Could you check a few things on this model? Use its own coordinates, in mm. A direction names the side the tool comes from. Coordinates: 2 decimals unless noted, no trailing zeros. Loops run counter-clockwise (first coordinate to the right, second up) from the corner with the lowest first, then second, coordinate; pieces in that order, holes last.
from build123d import *

# Parameters (mm, degrees)
SKETCH_2_W               = 1.2
SKETCH_2_H               = 0.55
CHAMFER_1_SIZE           = 1
FILLET_1_R               = 0.4
HOLE_WIZARD_1_D          = 3
HOLE_WIZARD_1_DEPTH      = 15
PATTERN_CIRCULAR_1_COUNT = 4
SKETCH_5_W               = 2.5
SKETCH_5_H               = 10
CHAMFER_2_SIZE           = 0.6
PATTERN_CIRCULAR_2_COUNT = 4


with BuildPart() as part:
    # Эскиз1 → Повернуть1 (revolve)
    with BuildSketch(Plane.XY):
        Polygon((0, 0), (0, 12.5), (-25, 12.5), (-25, 16), (-31, 16), (-31, 0), align=None)
    revolve(axis=Axis((0, 0, 0), (1, 0, 0)))

    # Эскиз2 → Вырез-Повернуть1 (revolve, cut)
    with BuildSketch(Plane.XY):
        with Locations((-3.4, 12.225)):
            Rectangle(SKETCH_2_W, SKETCH_2_H)
    revolve(axis=Axis((0, 0, 0), (-1, 0, 0)), mode=Mode.SUBTRACT)

    # Фаска1
    chamfer_1_edges = [part.edges().sort_by_distance(p)[0] for p in [
        (0, -12.5, 0),
    ]]
    chamfer(chamfer_1_edges, length=CHAMFER_1_SIZE)

    # Скругление1
    fillet_1_edges = [part.edges().sort_by_distance(p)[0] for p in [
        (-25, -12.5, 0),
    ]]
    fillet(fillet_1_edges, radius=FILLET_1_R)

    # Отверстие1
    with Locations(Plane(origin=(0, 0, 0), x_dir=(0, 0, -1), z_dir=(1, 0, 0))):
        with Locations((4.949747468, 4.949747468)):
            hole_wizard_1 = Hole(HOLE_WIZARD_1_D / 2, depth=HOLE_WIZARD_1_DEPTH)

    # Круговой массив1: Отверстие1 ×4 about axis
    pattern_circular_1_axis = Axis((0, 0, 0), (1, 0, 0))
    for i in range(1, PATTERN_CIRCULAR_1_COUNT):
        add(hole_wizard_1.rotate(pattern_circular_1_axis, i * 360 / PATTERN_CIRCULAR_1_COUNT), mode=Mode.SUBTRACT)

    # Эскиз5 → Вырез-Повернуть2 (revolve, cut)
    with BuildSketch(Plane.XY):
        with Locations((-1.25, 5)):
            Rectangle(SKETCH_5_W, SKETCH_5_H)
    revolve(axis=Axis((0, 0, 0), (-1, 0, 0)), mode=Mode.SUBTRACT)

    # Фаска2
    chamfer_2_edges = [part.edges().sort_by_distance(p)[0] for p in [
        (0, -10, 0),
    ]]
    chamfer(chamfer_2_edges, length=CHAMFER_2_SIZE)

    # Эскиз7 → Сверло под метчик  спиральное M31 (revolve, cut)
    with BuildSketch(Plane(origin=(-31, 0, -10), x_dir=(0, 0, 1), z_dir=(0, 1, 0))):
        Polygon((0, 0), (0, 20.946355475), (1.575, 20), (1.575, 0), align=None)
    hole_wizard_m31 = revolve(axis=Axis((-37.35, 0, -10), (1, 0, 0)), mode=Mode.SUBTRACT)

    # Круговой массив2: Сверло под метчик  спиральное M31 ×4 about axis
    pattern_circular_2_axis = Axis((0, 0, 0), (1, 0, 0))
    for i in range(1, PATTERN_CIRCULAR_2_COUNT):
        add(hole_wizard_m31.rotate(pattern_circular_2_axis, i * 360 / PATTERN_CIRCULAR_2_COUNT), mode=Mode.SUBTRACT)


solid = part.part
1) If I drill on L1, parallel to Z at x = -2, y = 0; L2, parallel to Z at x = -12.5, y = -7.5; L3, parallel to Z at x = -5.5, y = -4, over which ranges is the centre line in solid material (lowest first)?
2) Imagine slicing it at D-D on x = -3.5. List the corners of the cut face in (y, z) for me, plus the area to 3 significant figures.
3) We'd pull the mould along Z, two halves only. Please class faces 4 (the cylindrical face through (-8.84, 4.04, -6.14)), 5 (the cylindrical face through (-28.04, -3.47, -15.62)), 6 (the flat face through (0, -3.4, -10.2)): released by +Z, released by -Z, zero draft, split by the parting line, or undercut.
4) Imagine slicing it at C-C on y = -13.5. List the corners of the cut face in (x, z) for me, plus the area to 3 significant figures.
5) Imagine slicing it at A-A on x = -23. List the corners of the cut face in (y, z) for me (3 decimals), plus the area to 3 significant figures.
6) Imagine slicing it at B-B on x = -13. State how many separate pieces and enclosed holes the cut face has, plus the area to 3 significant figures.
7) Will these pins go through, and if not, where does the flat tip stop? pin 1 (1.5 mm diameter, centred on x = -5, z = -10.5, fed in from +Y); pin 2 (1 mm diameter, centred on x = -13.5, z = 0, fed in from -Y); pin 3 (1.5 mm diameter, centred on x = -7.5, z = -3.5, fed in from -Y).
8) For faces 1 (the flat face through (-2.5, 0, 0)), 2 (the flat face through (-31, 0, 0)), 3 (the cylindrical face through (-21.14, 11.25, 0.96)), which set-ups out of +Z, -Z, +X, -X, +Y, -Y let a thin tool reach every point of the face, with its end or its side?
Solved:
1. L1: z = -12.5 to -10, 10 to 12.5
1. L2: z = -10 to 10
1. L3: z = -11.84 to -6.11, -3.79 to 3.79, 6.11 to 11.84
2. outline: circle Ø23.9 at (0, 0); hole circle Ø3 at (-4.95, -4.95); hole circle Ø3 at (-4.95, 4.95); hole circle Ø3 at (4.95, -4.95); hole circle Ø3 at (4.95, 4.95)
2. area: 420 mm2
3. face 4: undercut
3. face 5: split by the parting line
3. face 6: zero draft
4. outline: (-31, -8.59) - (-25, -8.59) - (-25, 8.59) - (-31, 8.59) - close
4. area: 103 mm2
5. outline: circle Ø25 at (0, 0); hole circle Ø3.15 at (-10, 0); hole circle Ø3.15 at (0, -10); hole circle Ø3.15 at (0, 10); hole circle Ø3.15 at (10, 0)
5. area: 460 mm2
6. separate pieces: 1
6. enclosed holes: 8
6. area: 431 mm2
7. pin 1: stops at y = 7.82
7. pin 2: stops at y = -12.5
7. pin 3: stops at y = -12.19
8. face 1: +X
8. face 2: +Z, -Z, -X, +Y, -Y
8. face 3: -X
